For this review, take the finished solid that the model builds, in its own axes (mm). Give positions to 0.01 mm unless a question says otherwise; leave off trailing zeros. Order: outer loops, then holes, each group sorted by start corner. A loop starts at its lowest first (then second) coordinate and runs counter-clockwise, first axis right, second up. Notation, with made-up numbers: (-34.75, -0.5) - (17.25, -0.5) arc R20 cw to (17.25, 22.5) - close; hole circle Ø7 at (29, 8.5). An arc over 180 degrees is marked (long way). Use a Markdown table: item, result. Add a question column.
1) We need section B-B on y = -94. Write out the cut boundary in (x, z), then the cut area to 3 significant figures.
2) We need section A-A on x = 108.5. Write out the cut boundary in (y, z), then the cut area to 3 significant figures.
3) Wall thickness on L1, parallel to X at y = -46, z = 0.2; L2, parallel to Y at x = 29, z = 0.4: over which ranges is each line inside the solid? List them lowest first.
4) We need section C-C on z = 0.35. Write out the cut boundary in (x, y), then the cut area to 4 significant figures.
Autodesk Inventor part; units mm, degrees
ref_plane "YZ Plane" through (0, 0, 0) normal (1, 0, 0) x (0, 1, 0)
ref_plane "XZ Plane" through (0, 0, 0) normal (0, 1, 0) x (-1, 0, 0)
ref_plane "XY Plane" through (0, 0, 0) normal (0, 0, 1) x (1, 0, 0)
sketch "Sketch1" plane through (0, 0, 0) normal (0, 0, 1) x (1, 0, 0)
  line L0 (-150, -130) -> (150, -130)
  line L1 (150, -130) -> (150, 130)
  line L2 (150, 130) -> (-150, 130)
  line L3 (-150, 130) -> (-150, -130)
  line L4 (-150, -130) -> (150, 130) construction
  line L5 (150, -130) -> (-150, 130) construction
  point P0 (0, 0)
  dimension "d0" = 300
  dimension "d1" = 260
extrude "Plate1" add sketch "Sketch1" along normal blind 0.5
sketch "Sketch3" plane through (0, 0, 0.5) normal (0, 0, 1) x (1, 0, 0)
  line L0 (-140, -120) -> (140, -120)
  line L1 (140, -120) -> (140, 120)
  line L2 (140, 120) -> (-140, 120)
  line L3 (-140, 120) -> (-140, -120)
  line L4 (-140, -120) -> (140, 120) construction
  line L5 (140, -120) -> (-140, 120) construction
  line L6 (140, -120) -> (-10, -120)
  line L7 (-10, -120) -> (-10, -5)
  line L8 (-10, -5) -> (140, -5)
  line L9 (140, -5) -> (140, -120)
  point P0 (0, 0)
  dimension "d3" = 280
  dimension "d4" = 240
  dimension "d5" = 150
  dimension "d6" = 115
extrude "Cut1" cut sketch "Sketch3" against normal blind 0.5 contours L7 L8 L1 L0
sketch "Sketch4" plane through (0, 0, 0.5) normal (0, 0, 1) x (1, 0, 0)
  line L0 (-150, 130) -> (150, 130)
  point P0 (0, 0)
  dimension "d9" = 300
equation "\"d7\" = Thickness"
equation "\"BendRadius\" = Thickness"
equation "\"BendReliefWidth\" = Thickness"
equation "\"BendReliefDepth\" = 0.5 * Thickness"
equation "\"CornerReliefSize\" = 4 * Thickness"
equation "\"MinimumRemnant\" = 2 * Thickness"
equation "\"TransitionRadius\" = BendRadius"
equation "\"JacobiRadiusSize\" = BendRadius"
equation "\"GapSize\" = Thickness"
equation "\"d2\" = BendRadius"
properties part number "rightPanel"
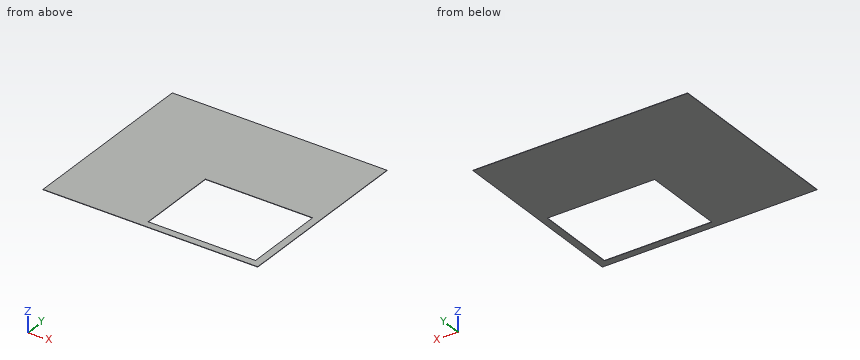
Checked values:
| question | item | result |
|---|---|---|
| 1 | outline | (-150, 0) - (-10, 0) - (-10, 0.5) - (-150, 0.5) - close; (140, 0) - (150, 0) - (150, 0.5) - (140, 0.5) - close |
| 1 | area | 75.0 mm² |
| 2 | outline | (-130, 0) - (-120, 0) - (-120, 0.5) - (-130, 0.5) - close; (-5, 0) - (130, 0) - (130, 0.5) - (-5, 0.5) - close |
| 2 | area | 72.5 mm² |
| 3 | L1 | -150 to -10, 140 to 150 |
| 3 | L2 | -130 to -120, -5 to 130 |
| 4 | outline | (-150, -130) - (150, -130) - (150, 130) - (-150, 130) - close; hole (-10, -120) - (140, -120) - (140, -5) - (-10, -5) - close |
| 4 | area | 60,750 mm² |
